```python
from build123d import *

# Parameters (mm, degrees)
SALIENTE_EXTRUIR1_DEPTH = 6


with BuildPart() as part:
    # Croquis1 → Saliente-Extruir1 (new body)
    with BuildSketch(Plane(origin=(0, 0, 0), x_dir=(1, 0, 0), z_dir=(0, 1, 0))):
        with BuildLine():
            Line((193.24437935, 2.559419019), (193.24437935, 12.559419019))
            Line((193.24437935, 12.559419019), (172.55, 12.559419019))
            Line((172.55, 12.559419019), (172.55, 6.059193777))
            ThreePointArc((172.55, 6.059193777), (173.474604635, 5.531104241), (173.840337631, 4.531098409))
            Line((173.840337631, 4.531098409), (173.840337631, 2.981098409))
            ThreePointArc((173.840337631, 2.981098409), (173.651640801, 2.239914437), (173.131494174, 1.679193777))
            Line((173.131494174, 1.679193777), (172.962249241, 1.679193777))
            ThreePointArc((172.962249241, 1.679193777), (171, 0.866183792), (169.037750759, 1.679193777))
            Line((169.037750759, 1.679193777), (168.868505826, 1.679193777))
            ThreePointArc((168.868505826, 1.679193777), (168.348359199, 2.239914437), (168.159662369, 2.981098409))
            Line((168.159662369, 2.981098409), (168.159662369, 4.531098409))
            ThreePointArc((168.159662369, 4.531098409), (168.525395365, 5.531104241), (169.45, 6.059193777))
            Line((169.45, 6.059193777), (169.45, 12.559419019))
            Line((169.45, 12.559419019), (152.1, 12.559419019))
            Line((152.1, 12.559419019), (149.6, 12.559419019))
            Line((149.6, 12.559419019), (149.6, 18.359419019))
            Line((149.6, 18.359419019), (134.6, 18.359419019))
            Line((134.6, 18.359419019), (134.6, 12.559419019))
            Line((134.6, 12.559419019), (132.1, 12.559419019))
            Line((132.1, 12.559419019), (85.25, 12.559419019))
            Line((85.25, 12.559419019), (85.25, 6.059193777))
            ThreePointArc((85.25, 6.059193777), (86.174604635, 5.531104241), (86.540337631, 4.531098409))
            Line((86.540337631, 4.531098409), (86.540337631, 2.981098409))
            ThreePointArc((86.540337631, 2.981098409), (86.351640801, 2.239914437), (85.831494174, 1.679193777))
            Line((85.831494174, 1.679193777), (85.662249241, 1.679193777))
            ThreePointArc((85.662249241, 1.679193777), (83.7, 0.866183792), (81.737750759, 1.679193777))
            Line((81.737750759, 1.679193777), (81.568505826, 1.679193777))
            ThreePointArc((81.568505826, 1.679193777), (81.048359199, 2.239914437), (80.859662369, 2.981098409))
            Line((80.859662369, 2.981098409), (80.859662369, 4.531098409))
            ThreePointArc((80.859662369, 4.531098409), (81.225395365, 5.531104241), (82.15, 6.059193777))
            Line((82.15, 6.059193777), (82.15, 12.559419019))
            Line((82.15, 12.559419019), (64.8, 12.559419019))
            Line((64.8, 12.559419019), (62.3, 12.559419019))
            Line((62.3, 12.559419019), (62.3, 18.359419019))
            Line((62.3, 18.359419019), (47.3, 18.359419019))
            Line((47.3, 18.359419019), (47.3, 12.559419019))
            Line((47.3, 12.559419019), (44.8, 12.559419019))
            Line((44.8, 12.559419019), (-2.05, 12.559419019))
            Line((-2.05, 12.559419019), (-2.05, 6.059193777))
            ThreePointArc((-2.05, 6.059193777), (-1.125395365, 5.531104241), (-0.759662369, 4.531098409))
            Line((-0.759662369, 4.531098409), (-0.759662369, 2.981098409))
            ThreePointArc((-0.759662369, 2.981098409), (-0.948359199, 2.239914437), (-1.468505826, 1.679193777))
            Line((-1.468505826, 1.679193777), (-1.637750759, 1.679193777))
            ThreePointArc((-1.637750759, 1.679193777), (-3.6, 0.866183792), (-5.562249241, 1.679193777))
            Line((-5.562249241, 1.679193777), (-5.731494174, 1.679193777))
            ThreePointArc((-5.731494174, 1.679193777), (-6.251640801, 2.239914437), (-6.440337631, 2.981098409))
            Line((-6.440337631, 2.981098409), (-6.440337631, 4.531098409))
            ThreePointArc((-6.440337631, 4.531098409), (-6.074604635, 5.531104241), (-5.15, 6.059193777))
            Line((-5.15, 6.059193777), (-5.15, 12.559419019))
            Line((-5.15, 12.559419019), (-22.5, 12.559419019))
            Line((-22.5, 12.559419019), (-25, 12.559419019))
            Line((-25, 12.559419019), (-25, 18.359419019))
            Line((-25, 18.359419019), (-40, 18.359419019))
            Line((-40, 18.359419019), (-40, 12.559419019))
            Line((-40, 12.559419019), (-42.5, 12.559419019))
            Line((-42.5, 12.559419019), (-42.5, 2.559419019))
            ThreePointArc((-42.5, 2.559419019), (-39.571067812, -4.511648793), (-32.5, -7.440580981))
            Line((-32.5, -7.440580981), (183.24437935, -7.440580981))
            ThreePointArc((183.24437935, -7.440580981), (190.315447162, -4.511648793), (193.24437935, 2.559419019))
        make_face()
    extrude(amount=SALIENTE_EXTRUIR1_DEPTH)


solid = part.part
```
Here's how the part is built. I have some questions about the finished solid (model axes, mm). A direction names the side the tool comes from. Coordinates: 2 decimals unless noted, no trailing zeros. Write each loop counter-clockwise with the first axis right and the second up, starting at its lowest first coordinate (ties: lowest second). Pieces come first, ordered by that corner, then holes. Notation, with made-up numbers: (5.25, -16) -> (59.25, -16) arc R22 cw to (59.25, 9) -> close; hole circle Ø2 at (45, -21.75). An arc over 180 degrees is marked (long way). Use a Markdown table: item, result. Add a question column.
(1) If we section it at A-A, the plane z = -10: Write out the boundary of the cut face in (x, y).
(2) Please list where these lines run through material, in increasing order: line 1 (X direction, y = 4.3, z = -6.25); line 2 (X direction, y = 2.05, z = -4.5); line 3 (X direction, y = 0.6, z = -12.75).
(3) If we section it at B-B, the plane x = 93: Write out the boundary of the cut face in (y, z).
(4) We'd pull the mould along X, two halves only. Please class faces 5 (the cylindrical face through (-39.65, 2.96, 4.43)), 6 (the flat face through (-2.05, 3, -9)), 7 (the flat face through (85.25, 3, -9)), 8 (the flat face through (142, 3, -18.359)): +X half, -X half, draft (parallel to the pull), parting line (faces both ways), or undercut.
(5) If we section it at C-C, the plane z = 4.5: Write out the boundary of the cut face in (x, y).
(6) For faces 1 (the flat face through (110, 3, -12.559)), 2 (the flat face through (-40, 3, -16)), 3 (the cylindrical face through (-3.569, 2.958, -0.866)), 4 (the flat face through (149.6, 3, -15)), which set-ups out of +Z, -Z, +X, -X, +Y, -Y let a thin tool reach every point of the face, with its end or its side?
(7) I'm going to push flat-ended pins straight in: P1, Ø3, axis at x = -14.5, y = 2, coming from the -Z side; P2, Ø1.7, axis at y = 2.5, z = -17, coming from the -X side; P3, Ø1.7, axis at y = 3.5, z = -14.5, coming from the +X side. Where does each tip first touch, or does it pass through?
Outcome:
| question | item | result |
|---|---|---|
| 1 | outline | (-42.5, 0) -> (-5.15, 0) -> (-5.15, 6) -> (-42.5, 6) -> close; (-2.05, 0) -> (82.15, 0) -> (82.15, 6) -> (-2.05, 6) -> close; (85.25, 0) -> (169.45, 0) -> (169.45, 6) -> (85.25, 6) -> close; (172.55, 0) -> (193.24, 0) -> (193.24, 6) -> (172.55, 6) -> close |
| 2 | line 1 | x = -42.5 to -5.15, -2.05 to 82.15, 85.25 to 169.45, 172.55 to 193.24 |
| 2 | line 2 | x = -42.5 to -6.44, -0.76 to 80.86, 86.54 to 168.16, 173.84 to 193.24 |
| 2 | line 3 | x = -40 to -25, 47.3 to 62.3, 134.6 to 149.6 |
| 3 | outline | (0, -12.56) -> (6, -12.56) -> (6, 7.44) -> (0, 7.44) -> close |
| 4 | face 5 | -X half |
| 4 | face 6 | undercut |
| 4 | face 7 | undercut |
| 4 | face 8 | draft |
| 5 | outline | (-39.58, 0) -> (190.33, 0) -> (190.33, 6) -> (-39.58, 6) -> close |
| 6 | face 1 | -Z, +Y, -Y |
| 6 | face 2 | -Z, -X, +Y, -Y |
| 6 | face 3 | +Y, -Y |
| 6 | face 4 | -Z, +X, +Y, -Y |
| 7 | P1 | stops at z = -12.56 |
| 7 | P2 | stops at x = -40 |
| 7 | P3 | stops at x = 149.6 |
